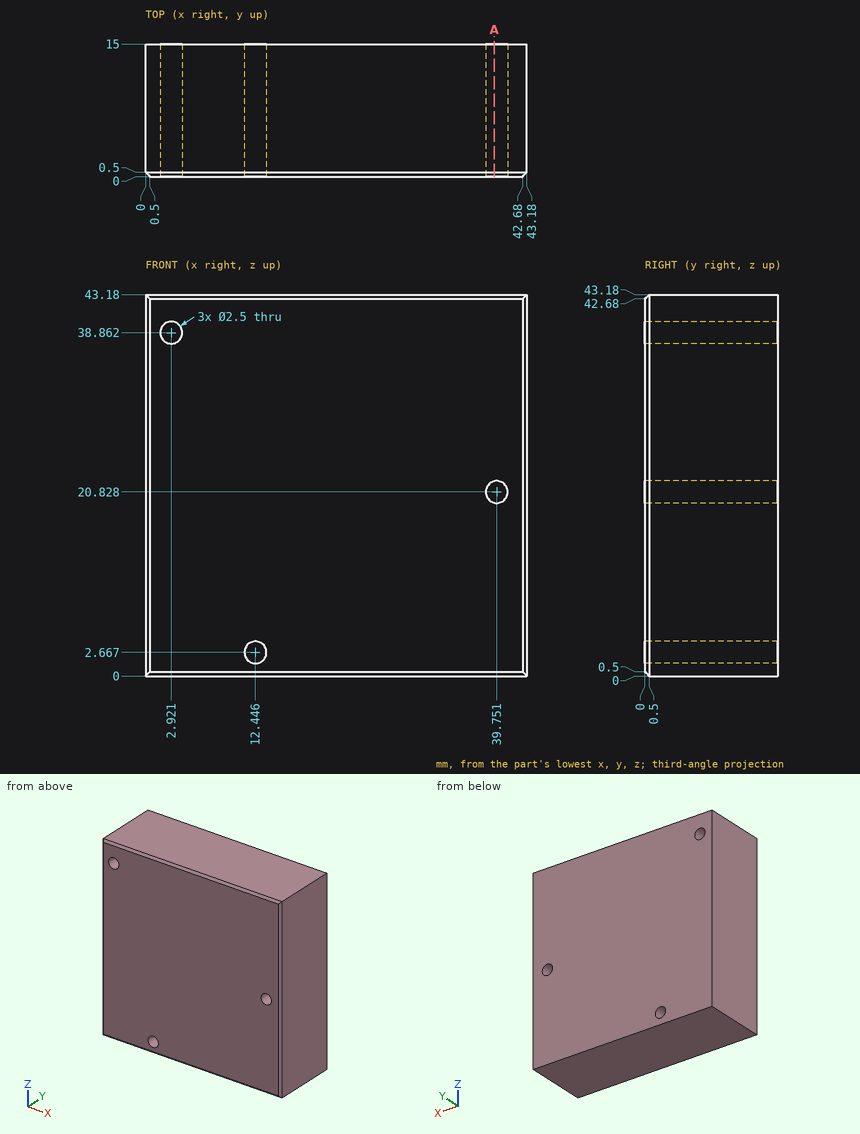
Verification items for this drawing (mm, ordinates from the low corner). Coordinates: 2 decimals unless noted, no trailing zeros. Write each loop counter-clockwise with the first axis right and the second up, starting at its lowest first coordinate (ties: lowest second). Pieces come first, ordered by that corner, then holes. Notation, with made-up numbers: M 82.5,-5 L 90.5,-5 A21 cw 90.5,26 Z; hole C 75.25,78.5 d4. An arc over 180 degrees is marked long. Answer as a JSON object with one key per item and string values. Group by question number.
(1) Cross-section at A-A, the plane x = 39.5. Record the cut outline in (y, z).
(2) Material ranges on line 1 (X direction, y = 4.5, z = 39); line 2 (X direction, y = 1.75, z = 3); line 3 (Z direction, x = 13.5, y = 6.75) (3 decimals), recorded low to high.
(3) Gauge pin test, flat end, axial feed: pin 1 (3 mm diameter, centred on x = 2.921, z = 38.862, fed in from +Y). Record the tip position at first contact, or that the pin passes through.
Reply:
{
 "1": {"outline": "M 0,0.5 L 0.5,0 L 15,0 L 15,19.6 L 0,19.6 Z; M 0,22.05 L 15,22.05 L 15,43.18 L 0.5,43.18 L 0,42.68 Z"},
 "2": {"line 1": "0 to 1.68, 4.16 to 43.18", "line 2": "0 to 11.24, 13.65 to 43.18", "line 3": "0 to 1.995, 3.339 to 43.18"},
 "3": {"pin 1": "y = 15"}
}
